Source: CAD feature listing. Evaluate the final solid. Frame: model axes, mm. A direction names the side the tool comes from. Round coordinates to 2 decimals unless told otherwise and drop trailing zeros. Loops run counter-clockwise (first coordinate to the right, second up) from the corner with the lowest first, then second, coordinate; pieces in that order, holes last. Notation, with made-up numbers: M 20.25,13.25 L 32.25,13.25 A27 cw 32.25,42.25 Z; hole C 12.25,23 d10. An arc over 180 degrees is marked long. Answer as a JSON object with one key per item and string values.
from build123d import *

# Parameters (mm, degrees)
F0_W     = 35
F0_H     = 10
F1_DEPTH = 13.8
F2_W     = 15
F2_H     = 10
F3_DEPTH = 8.8
F4_R     = 2
F5_DEPTH = 13.8


with BuildPart() as f1:
    # F0 (on Front) → F1 (new body)
    with BuildSketch(Plane.XZ):
        Rectangle(F0_W, F0_H)
    extrude(amount=F1_DEPTH)

    # F2 (on face) → F3 (cut)
    with BuildSketch(Plane.XZ.offset(13.8)):
        with Locations((-10, 0)):
            Rectangle(F2_W, F2_H)
    extrude(amount=-F3_DEPTH, mode=Mode.SUBTRACT)

    # F4 (on face) → F5 (cut)
    with BuildSketch(Plane.XZ.offset(13.8)):
        with Locations((2.5, 0)):
            Circle(F4_R)
        with Locations((11.5, 0)):
            Circle(F4_R)
    extrude(amount=-F5_DEPTH, mode=Mode.SUBTRACT)


solid = f1.part
Item 1: Line query: probe 1 along Z at (x, y) = (11.5, -10.25); probe 2 along X at (y, z) = (-12.5, 0.5); probe 3 along Y at (x, z) = (-13, -1.5). Output: solid intervals per line, ascending. Write a range as from..to.
Answer sheet:
{"probe 1": "z = -5..-2, 2..5", "probe 2": "x = -2.5..0.56, 4.44..9.56, 13.44..17.5", "probe 3": "y = -5..0"}
Item 2: Contact query for flat-ended pins moving along their axis: pin 1 Ø6 at (x, z) = (-3.5, -2) entering from -Y; pin 2 Ø5 at (y, z) = (-9, 0) entering from -X; pin 3 Ø5 at (x, z) = (-7, 0.5) entering from -Y. Output: stop coordinate, or through.
Answer sheet:
{"pin 1": "stops at y = -13.8", "pin 2": "stops at x = -2.5", "pin 3": "stops at y = -5"}
Item 3: Section D-D on z = -3.5. Return the cut outline in (x, y), then the cut area to 3 significant figures.
Answer sheet:
{"outline": "M -17.5,-5 L -2.5,-5 L -2.5,-13.8 L 17.5,-13.8 L 17.5,0 L -17.5,0 Z", "area": "351 mm²"}
Item 4: Section B-B on z = 0. Return the cut outline in (x, y).
Answer sheet:
{"outline": "M -17.5,-5 L -2.5,-5 L -2.5,-13.8 L 0.5,-13.8 L 0.5,0 L -17.5,0 Z; M 4.5,-13.8 L 9.5,-13.8 L 9.5,0 L 4.5,0 Z; M 13.5,-13.8 L 17.5,-13.8 L 17.5,0 L 13.5,0 Z"}
Item 5: Section A-A on y = -9.25. Return the cut outline in (x, z), then the cut area to 3 significant figures.
Answer sheet:
{"outline": "M -2.5,-5 L 17.5,-5 L 17.5,5 L -2.5,5 Z; hole C 2.5,0 d4; hole C 11.5,0 d4", "area": "175 mm²"}
Item 6: Section C-C on x = 11.5. Return the cut outline in (y, z), then the cut area to 3 significant figures.
Answer sheet:
{"outline": "M -13.8,-5 L 0,-5 L 0,-2 L -13.8,-2 Z; M -13.8,2 L 0,2 L 0,5 L -13.8,5 Z", "area": "82.8 mm²"}
Item 7: Access query for faces 1 (the flat face through (-2.5, -9, 0)), 2 (the flat face through (0, 0, 0)). Directions: +Z, -Z, +X, -X, +Y, -Y. A direction counts if a zero-diameter tool reaches every point of the face in a straight line with its end or side. Return the directions, or none.
Answer sheet:
{"face 1": "+Z, -Z, -X, -Y", "face 2": "+Z, -Z, +X, -X, +Y"}
